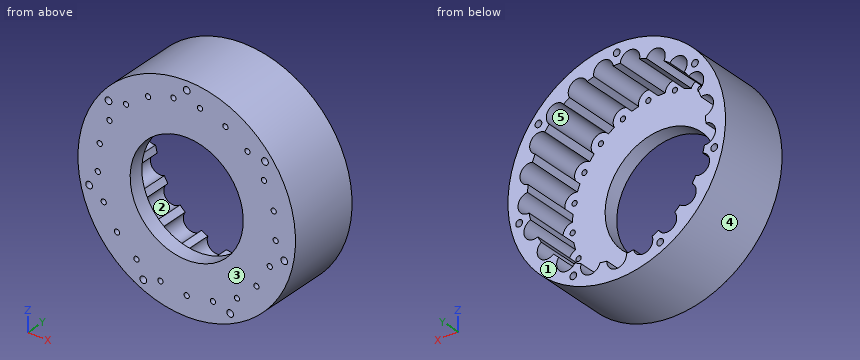
```python
from build123d import *

# Parameters (mm, degrees)
SKIZZE1_R                        = 50
AUFSATZ_LINEAR_AUSTRAGEN1_DEPTH  = 7
SKIZZE2_R                        = 50
SKIZZE2_R_2                      = 41
AUFSATZ_LINEAR_AUSTRAGEN2_DEPTH  = 27
SKIZZE3_R                        = 26
SCHNITT_LINEAR_AUSTRAGEN1_DEPTH  = 27
SKIZZE4_R                        = 4.5
SCHNITT_LINEAR_AUSTRAGEN2_DEPTH  = 27
KREISMUSTER1_COUNT               = 21
F_2_4_2_4_DURCHMESSER_BOHRUNG1_D = 2.4
KREISMUSTER2_COUNT               = 21
F_3_1_3_1_DURCHMESSER_BOHRUNG1_D = 3.1
KREISMUSTER3_COUNT               = 7


with BuildPart() as part:
    # Skizze1 → Aufsatz-Linear austragen1 (new body)
    with BuildSketch(Plane(origin=(0, 0, 0), x_dir=(1, 0, 0), z_dir=(0, 1, 0))):
        with Locations(Location((0, 0, 0), (0, 0, 270))):
            Circle(SKIZZE1_R)
    extrude(amount=AUFSATZ_LINEAR_AUSTRAGEN1_DEPTH)

    # Skizze2 → Aufsatz-Linear austragen2 (add)
    with BuildSketch(Plane(origin=(0, 7, 0), x_dir=(1, 0, 0), z_dir=(0, 1, 0))):
        with Locations(Location((0, 0, 0), (0, 0, 270))):
            Circle(SKIZZE2_R)
        with Locations(Location((0, 0, 0), (0, 0, 270))):
            Circle(SKIZZE2_R_2, mode=Mode.SUBTRACT)
    extrude(amount=AUFSATZ_LINEAR_AUSTRAGEN2_DEPTH)

    # Skizze3 → Schnitt-Linear austragen1 (cut)
    with BuildSketch(Plane(origin=(0, 7, 0), x_dir=(1, 0, 0), z_dir=(0, 1, 0))):
        with Locations(Location((0, 0, 0), (0, 0, 270))):
            Circle(SKIZZE3_R)
    extrude(amount=-SCHNITT_LINEAR_AUSTRAGEN1_DEPTH, mode=Mode.SUBTRACT)

    # Skizze4 → Schnitt-Linear austragen2 (cut)
    with BuildSketch(Plane(origin=(0, 34, 0), x_dir=(1, 0, 0), z_dir=(0, 1, 0))):
        with Locations((0, 41)):
            Circle(SKIZZE4_R)
    schnitt_linear_austragen2 = extrude(amount=-SCHNITT_LINEAR_AUSTRAGEN2_DEPTH, mode=Mode.SUBTRACT)

    # Kreismuster1: Schnitt-Linear austragen2 ×21 about axis
    kreismuster1_axis = Axis((0, 0, 0), (0, 1, 0))
    for i in range(1, KREISMUSTER1_COUNT):
        add(schnitt_linear_austragen2.rotate(kreismuster1_axis, i * 360 / KREISMUSTER1_COUNT), mode=Mode.SUBTRACT)

    # Ø2.4 (2.4) Durchmesser Bohrung1 (through all)
    with Locations(Plane(origin=(0, 7, 0), x_dir=(1, 0, 0), z_dir=(0, 1, 0))):
        with Locations((0, 41)):
            f_2_4_2_4_durchmesser_bohrung1 = Hole(F_2_4_2_4_DURCHMESSER_BOHRUNG1_D / 2)

    # Kreismuster2: Ø2.4 (2.4) Durchmesser Bohrung1 ×21 about axis
    kreismuster2_axis = Axis((0, 0, 0), (0, 1, 0))
    for i in range(1, KREISMUSTER2_COUNT):
        add(f_2_4_2_4_durchmesser_bohrung1.rotate(kreismuster2_axis, i * 360 / KREISMUSTER2_COUNT), mode=Mode.SUBTRACT)

    # Ø3.1 (3.1) Durchmesser Bohrung1 (through all)
    with Locations(Plane(origin=(0, 34, 0), x_dir=(1, 0, 0), z_dir=(0, 1, 0))):
        with Locations((0, -46)):
            f_3_1_3_1_durchmesser_bohrung1 = Hole(F_3_1_3_1_DURCHMESSER_BOHRUNG1_D / 2)

    # Kreismuster3: Ø3.1 (3.1) Durchmesser Bohrung1 ×7 about axis
    kreismuster3_axis = Axis((0, 0, 0), (0, 1, 0))
    for i in range(1, KREISMUSTER3_COUNT):
        add(f_3_1_3_1_durchmesser_bohrung1.rotate(kreismuster3_axis, i * 360 / KREISMUSTER3_COUNT), mode=Mode.SUBTRACT)


solid = part.part
```
Check sheet for the modelled part. Datum: model origin and axes. Units: mm. Face numbers are marked on the shaded views. A direction names the side the tool comes from. Give positions to 0.01 mm unless a question says otherwise; leave off trailing zeros. Loops run counter-clockwise (first coordinate to the right, second up) from the corner with the lowest first, then second, coordinate; pieces in that order, holes last. Notation, with made-up numbers: (86, -2) - (113, -2) arc R21 cw to (113, 16) - close; hole circle Ø11 at (-23.5, -0.5). An arc over 180 degrees is marked (long way). One line per question, with ' | ' between items. Start each with the question number.
1. Set-up check for the marked faces 1 and 2: record each of +Z, -Z, +X, -X, +Y, -Y from which the full face is reachable in a straight line by a thin tool's end or side.
2. Draft check along X on the marked faces 3, 4 and 5. Enter one of: released by +X, released by -X, zero draft, split by the parting line, or undercut.
3. Cross-section at B-B, the plane y = 4. Give the number of separate pieces and of enclosed holes in the cut face, plus the area to 3 significant figures.
4. Gauge pin test, flat ends, axial feed: pin 1 Ø3 at (y, z) = (26.5, -22) entering from -X; pin 2 Ø2 at (x, y) = (-8.5, 14.5) entering from +Z; pin 3 Ø3 at (x, z) = (38.17, -14.98) entering from -Y; pin 4 Ø1.4 at (x, z) = (-39.97, 9.12) entering from -Y. Record the tip position at first contact, or that the pin passes through.
5. Cross-section at A-A, the plane x = 0. Enter the section's corners in (y, z), plus the area to 3 significant figures.
6. Cross-section at C-C, the plane z = 0. Enter the section's corners in (x, y).
7. Material ranges on line 1 along X through (y, z) = (1.5, 0); line 2 along X through (y, z) = (32, 40.5); line 3 along Z through (x, y) = (32, 14.5), recorded low to high. Write a range as [from, to].
Check result:
1) face 1: +Z, -Z, +X, -X, +Y | face 2: +Y
2) face 3: zero draft | face 4: split by the parting line | face 5: undercut
3) separate pieces: 1 | enclosed holes: 29 | area: 5,580 mm2
4) pin 1: stops at x = -45.6 | pin 2: stops at z = 49.43 | pin 3: stops at y = 0 | pin 4: passes through
5) outline: (0, -50) - (34, -50) - (34, -45.5) - (7, -45.5) - (7, -42.2) - (0, -42.2) - close; (0, -39.8) - (7, -39.8) - (7, -26) - (0, -26) - close; (0, 26) - (7, 26) - (7, 41) - (34, 41) - (34, 44.45) - (0, 44.45) - close; (0, 47.55) - (34, 47.55) - (34, 50) - (0, 50) - close | area: 578 mm2
6) outline: (-50, 0) - (-26, 0) - (-26, 7) - (-44.18, 7) - (-44.18, 34) - (-50, 34) - close; (26, 0) - (50, 0) - (50, 34) - (44.18, 34) - (44.18, 7) - (26, 7) - close
7) line 1: x = [-50, -26], [26, 50] | line 2: x = [-29.32, -20.54], [-15.04, -10.61], [10.61, 15.04], [20.54, 29.32] | line 3: z = [-38.42, -30.06], [25.63, 28.23], [31.88, 38.42]
